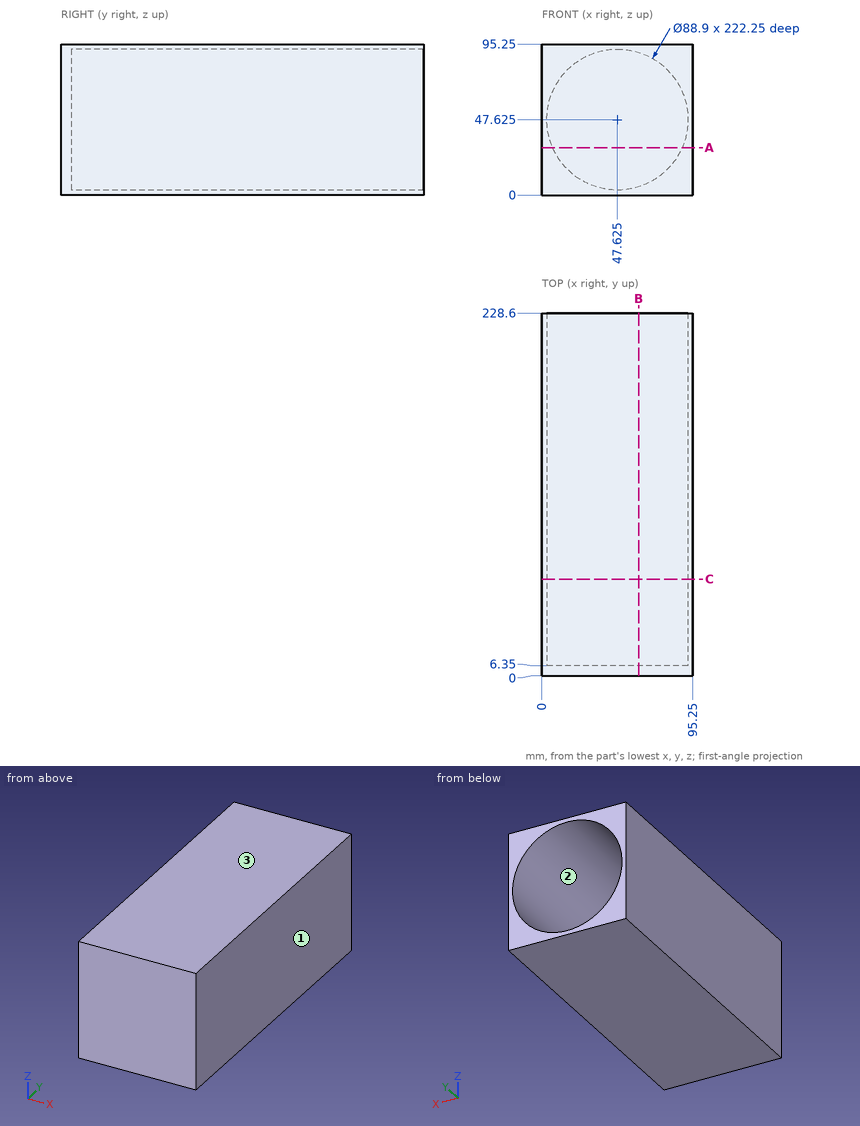
Design review of the part shown in the three views and the two pictorial views. Dimensions are in mm from the part's minimum x, y and z. Coordinates: 2 decimals unless noted, no trailing zeros. Loops run counter-clockwise (first coordinate to the right, second up) from the corner with the lowest first, then second, coordinate; pieces in that order, holes last. Notation, with made-up numbers: (15, 15) -> (60, 15) arc R13 ccw to (60, 19) -> close; hole circle Ø2 at (60.25, 22). An arc over 180 degrees is marked (long way). Answer as CSV lines item,"result".
Item 1: Take a section at A-A, the plane z = 30. State the section outline as (x, y) points.
Results below:
outline,"(0, 0) -> (95.25, 0) -> (95.25, 228.6) -> (88.43, 228.6) -> (88.43, 6.35) -> (6.82, 6.35) -> (6.82, 228.6) -> (0, 228.6) -> close"
Item 2: Take a section at C-C, the plane y = 61. State the section outline as (x, z) points (3 decimals), and give its area (3 significant figures).
Results below:
outline,"(0, 0) -> (95.25, 0) -> (95.25, 95.25) -> (0, 95.25) -> close; hole circle Ø88.9 at (47.625, 47.625)"
area,"2,870 mm2"
Item 3: For L1, parallel to Y at x = 70.5, z = 76; L2, parallel to X at y = 89.5, z = 28.5; L3, parallel to Z at x = 9, y = 70, list the stretches that pass through material, from the lowest coordinate up.
Results below:
L1,"y = 0 to 6.35"
L2,"x = 0 to 7.5, 87.75 to 95.25"
L3,"z = 0 to 25.63, 69.62 to 95.25"
Item 4: Draft analysis for pull direction Z (two halves, no side actions). For the marked faces 1, 2 and 3, state which applies: +Z half, -Z half, draft (parallel to the pull), parting line (faces both ways), or undercut.
Results below:
face 1,"draft"
face 2,"undercut"
face 3,"+Z half"
Item 5: Take a section at B-B, the plane x = 61. State the section outline as (y, z) points (3 decimals).
Results below:
outline,"(0, 0) -> (228.6, 0) -> (228.6, 5.235) -> (6.35, 5.235) -> (6.35, 90.015) -> (228.6, 90.015) -> (228.6, 95.25) -> (0, 95.25) -> close"
Item 6: Insertion check: pin 1 (8 mm diameter, centred on x = 81, z = 37.5, fed in from +Y). The pin has a flat end and moves straight along its axis. Give the tip position at first contact, or say it passes through.
Results below:
pin 1,"stops at y = 6.35"
